from build123d import *

# Parameters (mm, degrees)
SKETCH1_W                = 25.5
SKETCH1_H                = 21.2
BOSS_EXTRUDE1_DEPTH      = 16.2
SKETCH3_W                = 30.5
SKETCH3_H                = 25.6
BOSS_EXTRUDE2_DEPTH      = 2
BOSS_EXTRUDE3_DEPTH      = 9.25
BOSS_EXTRUDE4_DEPTH      = 0.5
BOSS_EXTRUDE4_DEPTH_BACK = 11.5
SKETCH6_R                = 0.75
CUT_EXTRUDE1_DEPTH       = 37.291080171
CUT_EXTRUDE1_DEPTH_BACK  = 37.291080171
SKETCH7_W                = 10
SKETCH7_H                = 10.2
BOSS_EXTRUDE5_DEPTH      = 0.5
BOSS_EXTRUDE6_DEPTH      = 9


with BuildPart() as part:
    # Sketch1 → Boss-Extrude1 (new body)
    with BuildSketch(Plane(origin=(0, 0, 0), x_dir=(1, 0, 0), z_dir=(0, 1, 0))):
        Rectangle(SKETCH1_W, SKETCH1_H)
    extrude(amount=BOSS_EXTRUDE1_DEPTH)

    # Sketch3 → Boss-Extrude2 (add)
    with BuildSketch(Plane(origin=(0, 16.2, 0), x_dir=(1, 0, 0), z_dir=(0, 1, 0))):
        Rectangle(SKETCH3_W, SKETCH3_H)
    extrude(amount=BOSS_EXTRUDE2_DEPTH)

    # Sketch4 → Boss-Extrude3 (add, symmetric)
    with BuildSketch(Plane.XY):
        with BuildLine():
            Line((-12.05, 18.2), (12.05, 18.2))
            ThreePointArc((12.05, 18.2), (11.927434436, 18.551874053), (11.79459622, 18.9))
            ThreePointArc((11.79459622, 18.9), (2.343455936, 20.945857513), (-6.340544141, 25.2))
            ThreePointArc((-6.340544141, 25.2), (-9.838853005, 22.224928134), (-12.05, 18.2))
        make_face()
    extrude(amount=BOSS_EXTRUDE3_DEPTH, both=True)

    # Sketch6 → Boss-Extrude4 (add, two sides: drawn at the far end of the back side and taken through both)
    # profile 1 of 2: a face of its own
    with BuildSketch(Plane(origin=(0, 0, 0), x_dir=(0, 0, -1), z_dir=(1, 0, 0)).offset(-BOSS_EXTRUDE4_DEPTH_BACK)):
        Polygon((-8.4, 0), (-8.4, -9.2), (-7.4, -10.2), (-3.1, -10.2), (-2.1, -9.2), (-2.1, 0), align=None)
        with Locations((-5.25, -7.05)):
            Circle(SKETCH6_R, mode=Mode.SUBTRACT)
    # profile 2 of 2: a face of its own
    with BuildSketch(Plane(origin=(0, 0, 0), x_dir=(0, 0, -1), z_dir=(1, 0, 0)).offset(-BOSS_EXTRUDE4_DEPTH_BACK)):
        Polygon((2.1, -9.2), (2.1, 0), (8.4, 0), (8.4, -9.2), (7.4, -10.2), (3.1, -10.2), align=None)
        with Locations(Location((5.25, -7.05, 0), (0, 0, 180))):
            Circle(SKETCH6_R, mode=Mode.SUBTRACT)
    extrude(amount=BOSS_EXTRUDE4_DEPTH + BOSS_EXTRUDE4_DEPTH_BACK)

    # Sketch7 → Cut-Extrude1 (cut, two sides: drawn at the far end of the back side and taken through both)
    with BuildSketch(Plane.XY.offset(8.4).offset(-CUT_EXTRUDE1_DEPTH_BACK)):
        with Locations((-5.5, -5.1)):
            Rectangle(SKETCH7_W, SKETCH7_H)
    extrude(amount=CUT_EXTRUDE1_DEPTH + CUT_EXTRUDE1_DEPTH_BACK, mode=Mode.SUBTRACT)

    # Sketch8 → Boss-Extrude5 (add, symmetric)
    with BuildSketch(Plane.XY):
        with BuildLine():
            Line((-12.75, 0), (12.75, 0))
            Line((12.75, 0), (12.75, -9.2))
            ThreePointArc((12.75, -9.2), (12.457106781, -9.907106781), (11.75, -10.2))
            Line((11.75, -10.2), (-11.75, -10.2))
            ThreePointArc((-11.75, -10.2), (-12.457106781, -9.907106781), (-12.75, -9.2))
            Line((-12.75, -9.2), (-12.75, 0))
        make_face()
    extrude(amount=BOSS_EXTRUDE5_DEPTH, both=True)

    # Sketch9 → Boss-Extrude6 (add, symmetric)
    with BuildSketch(Plane.XY):
        Polygon((-16.45, 15.5), (-14.75, 15.5), (-14.75, 10.5), (-12.75, 4.985823609), (-12.75, 0), (-16.45, 10.201226322), align=None)
        Polygon((12.75, 0), (16.45, 10.201226322), (16.45, 15.5), (14.75, 15.5), (14.75, 10.5), (12.75, 4.985823609), align=None)
    extrude(amount=BOSS_EXTRUDE6_DEPTH, both=True)


solid = part.part
Source: CAD feature listing. Evaluate the final solid. Frame: model axes, mm. A direction names the side the tool comes from. Give positions to 0.01 mm unless a question says otherwise; leave off trailing zeros. Order: outer loops, then holes, each group sorted by start corner. A loop starts at its lowest first (then second) coordinate and runs counter-clockwise, first axis right, second up. Notation, with made-up numbers: (-23, 13.5) -> (-8, 13.5) arc R12 cw to (-8, 33.5) -> close; hole circle Ø3 at (17.5, 3.25). An arc over 180 degrees is marked (long way). Write item = value, one per line.
Q1. Cut plane A-A, the plane y = 12. Output: boundary loops of the cut face in (x, z).
Data:
outline = (-16.45, -9) -> (-14.75, -9) -> (-14.75, 9) -> (-16.45, 9) -> close; (-12.75, -10.6) -> (12.75, -10.6) -> (12.75, 10.6) -> (-12.75, 10.6) -> close; (14.75, -9) -> (16.45, -9) -> (16.45, 9) -> (14.75, 9) -> close
Q2. Cut plane C-C, the plane y = -7.05. State how many separate pieces and enclosed holes the cut face has, and give its area (3 significant figures).
Data:
separate_pieces = 9
enclosed_holes = 0
area = 44.7 mm^2
Q3. Cut plane D-D, the plane x = 8. Output: boundary loops of the cut face in (y, z), and give its area (3 significant figures).
Data:
outline = (-10.2, -0.5) -> (0, -0.5) -> (0, -10.6) -> (16.2, -10.6) -> (16.2, -12.8) -> (18.2, -12.8) -> (18.2, -9.25) -> (19.43, -9.25) -> (19.43, 9.25) -> (18.2, 9.25) -> (18.2, 12.8) -> (16.2, 12.8) -> (16.2, 10.6) -> (0, 10.6) -> (0, 0.5) -> (-10.2, 0.5) -> close
area = 428 mm^2
Q4. Pull-direction query (X, two-part tool) for faces 1 (the face through (-11, -9.7, -7.9)), 2 (the face through (3, 0, -6)), 3 (the face through (-11.5, -5, -5)); classes: released by +X, released by -X, zero draft, split by the parting line, or undercut.
Data:
face_1 = zero draft
face_2 = undercut
face_3 = released by -X
Q5. Pin query (flat end, axial travel): pin 1 (6 mm diameter, centred on x = 1.5, y = 1, fed in from -Z); pin 2 (3 mm diameter, centred on y = -7, z = 6.5, fed in from -X); pin 3 (3 mm diameter, centred on y = -3, z = 6, fed in from +X). Return the tip coordinate at first contact, or that it passes through.
Data:
pin_1 = -10.6
pin_2 = -11.5
pin_3 = 0.5
Q6. Cut plane B-B, the plane z = 1.25. Output: boundary loops of the cut face in (x, y), and give its area (3 significant figures).
Data:
outline = (-16.45, 10.2) -> (-12.75, 0) -> (12.75, 0) -> (16.45, 10.2) -> (16.45, 15.5) -> (14.75, 15.5) -> (14.75, 10.5) -> (12.75, 4.99) -> (12.75, 16.2) -> (15.25, 16.2) -> (15.25, 18.2) -> (12.05, 18.2) arc R12.7 ccw to (11.79, 18.9) arc R40 cw to (-6.34, 25.2) arc R12.7 ccw to (-12.05, 18.2) -> (-15.25, 18.2) -> (-15.25, 16.2) -> (-12.75, 16.2) -> (-12.75, 4.99) -> (-14.75, 10.5) -> (-14.75, 15.5) -> (-16.45, 15.5) -> close
area = 600 mm^2
Q7. Set-up query: faces 4 (the face through (15.25, 17, 0)), 5 (the face through (-11, -5, -2.1)), 6 (the face through (16, 15.5, 0)). Return all of +Z, -Z, +X, -X, +Y, -Y with unobstructed straight access to the full face (end or side cutting, diameter ignored); none if empty.
Data:
face_4 = +Z, -Z, +X, +Y
face_5 = +X, -X, -Y
face_6 = +Z, -Z, +X
Q8. Material intervals for line 1 (Z direction, x = -11, y = -7.05); line 2 (X direction, y = 10.5, z = -8.25); line 3 (X direction, y = -7.5, z = 4), sorted ascending. Write a range as from..to.
Data:
line_1 = -8.4..-6, -4.5..-2.1, -0.5..0.5, 2.1..4.5, 6..8.4
line_2 = -16.45..-14.75, -12.75..12.75, 14.75..16.45
line_3 = -11.5..-10.5, -0.5..0.5
